```python
from build123d import *

# Parameters (mm, degrees)
F0_W     = 20
F0_H     = 55
F1_DEPTH = 35
F2_W     = 5
F2_H     = 20
F3_DEPTH = 35.001
F4_R     = 2.49999


# Not quite as in the source:
# - a fillet or chamfer is up to 0.001 mm smaller than in the source, because OpenCascade refuses the exact size


with BuildPart() as f1:
    # F0 (on Top) → F1 (new body)
    with BuildSketch(Plane.XY):
        Rectangle(F0_W, F0_H)
    extrude(amount=F1_DEPTH)

    # F2 (on face) → F3 (cut, through all)
    with BuildSketch(Plane.XY.offset(35)):
        Rectangle(F2_W, F2_H)
    extrude(amount=-F3_DEPTH, mode=Mode.SUBTRACT)

    # F4 (radius 2.5 in the source; OpenCascade refuses exactly that, so slightly less here)
    f4_edges = [f1.edges().sort_by_distance(p)[0] for p in [
        (-2.5, 10, 17.5),
        (2.5, 10, 17.5),
        (2.5, -10, 17.5),
        (-2.5, -10, 17.5),
    ]]
    fillet(f4_edges, radius=F4_R)


solid = f1.part
```
CAD build for the part. Positions are in the model's coordinates, mm. A direction names the side the tool comes from. Give positions to 0.01 mm unless a question says otherwise; leave off trailing zeros. Order: outer loops, then holes, each group sorted by start corner. A loop starts at its lowest first (then second) coordinate and runs counter-clockwise, first axis right, second up.
(1) Tool access for faces 1 (the flat face through (10, 0, 17)), 2 (the cylindrical face through (-2, -9, 17)): list every direction of +Z, -Z, +X, -X, +Y, -Y with a clear straight run to the whole face (end or side of a thin tool).
(2) Saw through at A-A, the plane y = 4. Give the cut face in (x, z), then the cut area to 3 significant figures.
(3) Drill centre lines: L1, parallel to X at y = -7, z = 27.5; L2, parallel to Y at x = 0.5, z = 6.5; L3, parallel to Y at x = -1.25, z = 4. Where is each one in solid material? Low to high.
(4) Mould opens along X. For faces 3 (the flat face through (-10, 0, 17)), 4 (the flat face through (0, 27.5, 17)), 5 (the cylindrical face through (-2, 9, 17)) say: released by +X, released by -X, zero draft, split by the parting line, or undercut.
(5) Saw through at C-C, the plane x = -1.5. Give the cut face in (y, z), then the cut area to 3 significant figures.
Results found:
1. face 1: +Z, -Z, +X, +Y, -Y
1. face 2: +Z, -Z
2. outline: (-10, 0) - (-2.5, 0) - (-2.5, 35) - (-10, 35) - close; (2.5, 0) - (10, 0) - (10, 35) - (2.5, 35) - close
2. area: 525 mm2
3. L1: x = -10 to -2.5, 2.5 to 10
3. L2: y = -27.5 to -9.95, 9.95 to 27.5
3. L3: y = -27.5 to -9.67, 9.67 to 27.5
4. face 3: released by -X
4. face 4: zero draft
4. face 5: undercut
5. outline: (-27.5, 0) - (-9.5, 0) - (-9.5, 35) - (-27.5, 35) - close; (9.5, 0) - (27.5, 0) - (27.5, 35) - (9.5, 35) - close
5. area: 1,260 mm2
